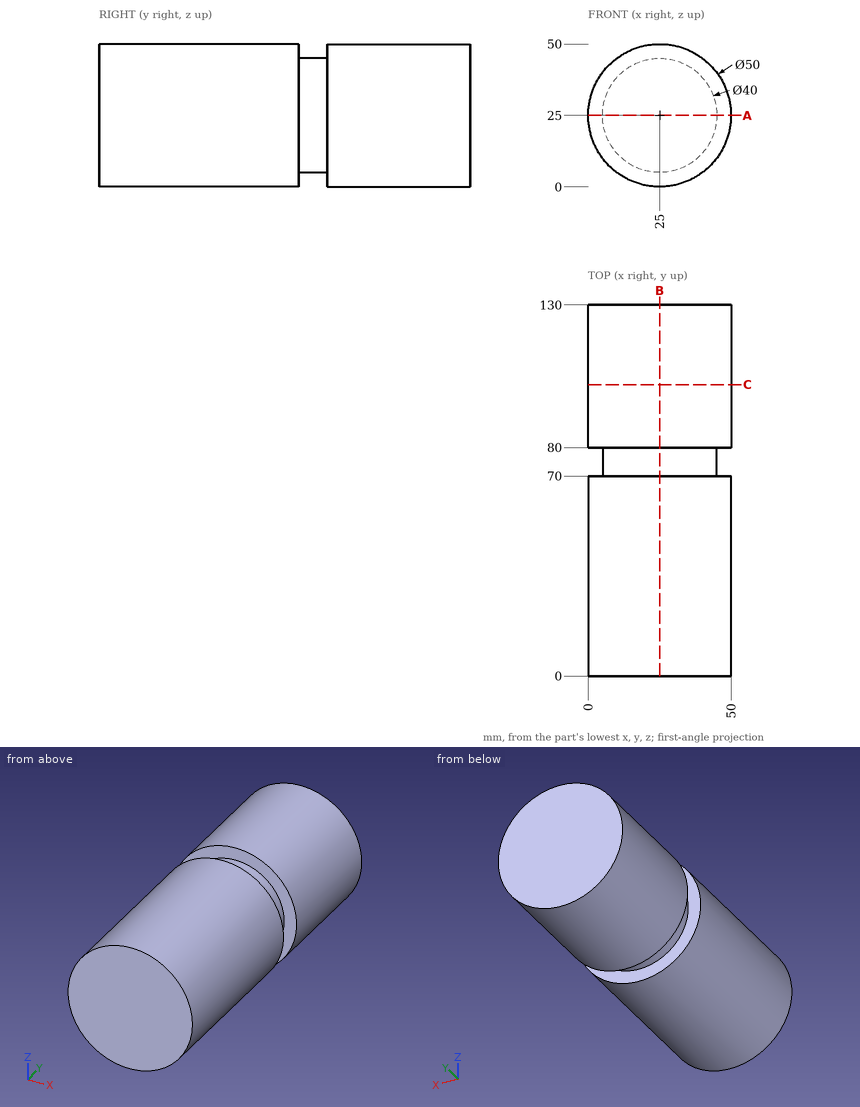
The drawing under review shows one solid part. Ordinate dimensions are in mm from its lowest x, y, z. Coordinates: 2 decimals unless noted, no trailing zeros. Write each loop counter-clockwise with the first axis right and the second up, starting at its lowest first coordinate (ties: lowest second). Pieces come first, ordered by that corner, then holes.
1) To check wall thickness, follow L1, parallel to Y at x = 3, z = 26; L2, parallel to X at y = 32, z = 40; L3, parallel to X at y = 124.5, z = 13. State the ranges of each line that lie inside material, in increasing order.
2) Add section B-B (x = 25). Write out the cut boundary in (y, z).
3) Insertion check: pin 1 (1 mm diameter, centred on y = 19.5, z = 23.5, fed in from -X); pin 2 (6 mm diameter, centred on y = 39.5, z = 39, fed in from +X); pin 3 (12 mm diameter, centred on x = 11.5, y = 104, fed in from +Z). Each pin has a flat end and moves straight along its axis. Give the tip position at first contact, or say it passes through.
4) Add section A-A (z = 25). Write out the cut boundary in (x, y), plus the area to 3 significant figures.
5) Add section C-C (y = 102). Write out the cut boundary in (x, z), plus the area to 3 significant figures.
Check result:
1. L1: y = 0 to 70, 80 to 130
1. L2: x = 5 to 45
1. L3: x = 3.07 to 46.93
2. outline: (0, 0) - (70, 0) - (70, 5) - (80, 5) - (80, 0) - (130, 0) - (130, 50) - (80, 50) - (80, 45) - (70, 45) - (70, 50) - (0, 50) - close
3. pin 1: stops at x = 0.02
3. pin 2: stops at x = 47.45
3. pin 3: stops at z = 48.85
4. outline: (0, 0) - (50, 0) - (50, 70) - (45, 70) - (45, 80) - (50, 80) - (50, 130) - (0, 130) - (0, 80) - (5, 80) - (5, 70) - (0, 70) - close
4. area: 6,400 mm2
5. outline: circle Ø50 at (25, 25)
5. area: 1,960 mm2
